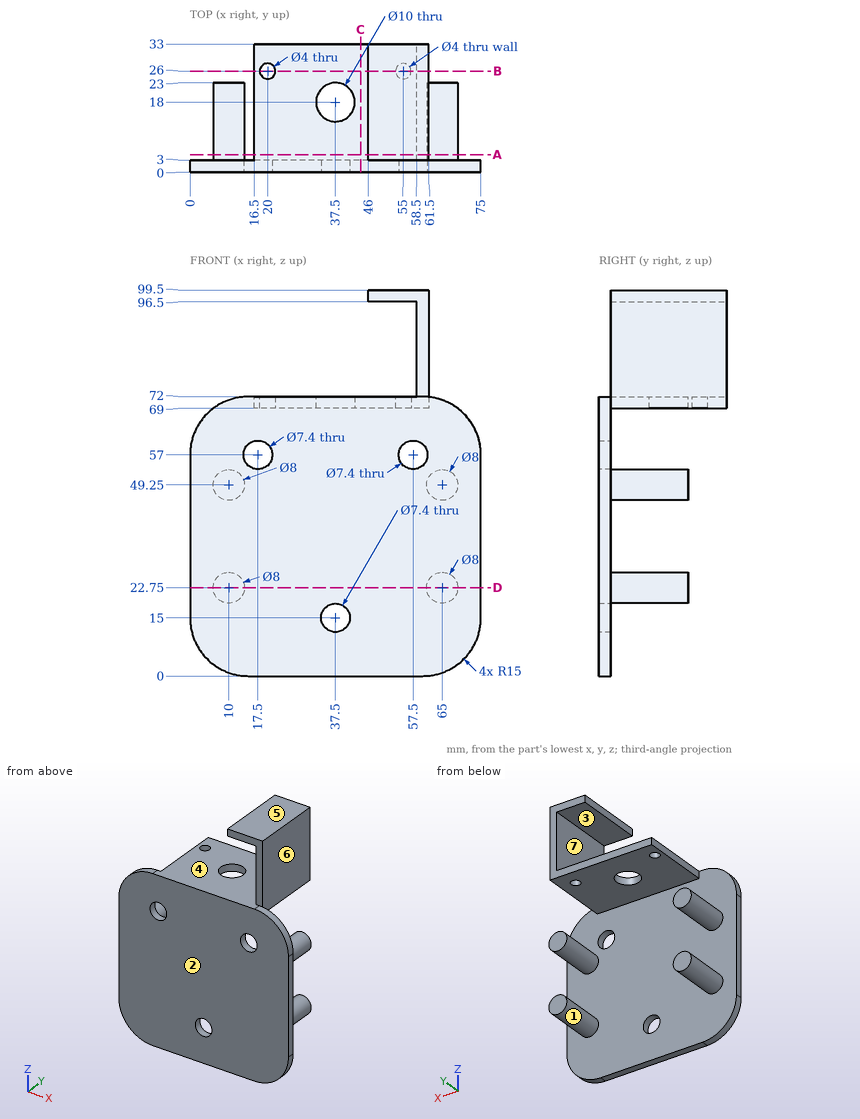
Study the drawing (mm; zero at the part's minimum x, y, z) and answer. A direction names the side the tool comes from. Round coordinates to 2 decimals unless told otherwise and drop trailing zeros. Loops run counter-clockwise (first coordinate to the right, second up) from the corner with the lowest first, then second, coordinate; pieces in that order, holes last. Notation, with made-up numbers: (20.25, -35.5) -> (79.25, -35.5) arc R13 ccw to (79.25, -21.5) -> close; hole circle Ø9 at (46, 80.25). An arc over 180 degrees is marked (long way). Write each question's results on one line, items separated by ' | '. Start each with the question number.
1. A tool of negligible diameter and unlimited length cuts with its end or side. For the marked faces 1, 2 and 3, from which of +Z, -Z, +X, -X, +Y, -Y can it reach the whole face along a straight path? Write none if from no direction.
2. Given pin 1 Ø10 at (y, z) = (7.5, 36) entering from +X; pin 2 Ø6 at (x, y) = (19, 10.5) entering from -Z; pin 3 Ø1.5 at (y, z) = (9, 22) entering from -X; pin 4 Ø3.5 at (y, z) = (14, 98.5) entering from -X, each flat-ended and moving along its own axis, determine where each tip first touches the part or whether it passes through.
3. Find the intervals of material crossed by probe 1 along Z at (x, y) = (55.5, 24); probe 2 along Y at (x, z) = (57.5, 7); probe 3 along Z at (x, y) = (60.5, 30), in increasing order. Write a range as from..to.
4. Section C-C (x = 44) is taken. Determine the outline of the cut face in (y, z), plus the area to 3 significant figures.
5. For a pull along Z with two mould halves and no side action, classify the marked faces 4, 5, 6 and 7 as +Z half, -Z half, draft (parallel to the pull), parting line (faces both ways), or undercut.
6. Section A-A (y = 4.5) is taken. Determine the outline of the cut face in (x, z).
7. Section B-B (y = 26) is taken. Determine the outline of the cut face in (x, z).
8. Section D-D (z = 22.75) is taken. Determine the outline of the cut face in (x, y).
Evaluation:
1) face 1: +Y | face 2: +Z, -Z, +X, -X, -Y | face 3: -X, +Y, -Y
2) pin 1: stops at x = 75 | pin 2: stops at z = 69 | pin 3: stops at x = 6 | pin 4: stops at x = 46
3) probe 1: z = 69..72, 96.5..99.5 | probe 2: y = 0..3 | probe 3: z = 69..99.5
4) outline: (0, 0) -> (3, 0) -> (3, 69) -> (33, 69) -> (33, 72) -> (0, 72) -> close | area: 306 mm2
5) face 4: undercut | face 5: +Z half | face 6: draft | face 7: undercut
6) outline: circle Ø8 at (10, 22.75); circle Ø8 at (10, 49.25); (16.5, 69) -> (61.5, 69) -> (61.5, 99.5) -> (46, 99.5) -> (46, 96.5) -> (58.5, 96.5) -> (58.5, 72) -> (16.5, 72) -> close; circle Ø8 at (65, 22.75); circle Ø8 at (65, 49.25)
7) outline: (16.5, 69) -> (18, 69) -> (18, 72) -> (16.5, 72) -> close; (22, 69) -> (53, 69) -> (53, 72) -> (22, 72) -> close; (46, 96.5) -> (58.5, 96.5) -> (58.5, 72) -> (57, 72) -> (57, 69) -> (61.5, 69) -> (61.5, 99.5) -> (46, 99.5) -> close
8) outline: (0, 0) -> (75, 0) -> (75, 3) -> (69, 3) -> (69, 23) -> (61, 23) -> (61, 3) -> (14, 3) -> (14, 23) -> (6, 23) -> (6, 3) -> (0, 3) -> close
